Verification items for the finished model (mm, model axes). Face numbers are marked on the shaded views. A direction names the side the tool comes from. Give positions to 0.01 mm unless a question says otherwise; leave off trailing zeros. Order: outer loops, then holes, each group sorted by start corner. A loop starts at its lowest first (then second) coordinate and runs counter-clockwise, first axis right, second up. Notation, with made-up numbers: (-15.75, 32.25) -> (18.25, 32.25) arc R12 cw to (18.25, 39.25) -> close; hole circle Ø2 at (-7.5, -37.75). An arc over 180 degrees is marked (long way). Write each question's results on one line, items separated by ' | '. Start each with the question number.
1. Set-up check for the marked faces 1, 2 and 3: record each of +Z, -Z, +X, -X, +Y, -Y from which the full face is reachable in a straight line by a thin tool's end or side.
2. Cross-section at B-B, the plane x = 0. Enter the section's corners in (y, z).
3. Cross-section at D-D, the plane x = -7.25. Enter the section's corners in (y, z).
4. Depth check by flat-ended pin: pin 1 Ø1.2 at (x, z) = (-5.5, -3.5) entering from +Y; pin 2 Ø4 at (x, y) = (2, 0.5) entering from -Z; pin 3 Ø1 at (x, z) = (-1, -5) entering from -Y. Enter the tip coordinate at first touch or a pass-through.
5. Cross-section at A-A, the plane y = 0. Enter the section's corners in (x, z), then the cut area to 3 significant figures.
6. Mould release check, pull along X, two halves, no side actions. Record for the marked faces 4, 5 and 6: +X half, -X half, draft (parallel to the pull), parting line (faces both ways), or undercut.
7. Material ranges on L1, parallel to Z at x = 7.25, y = -3; L2, parallel to Y at x = -1.75, z = -7.5; L3, parallel to X at y = 0, z = -2.25, recorded low to high. Write a range as from..to.
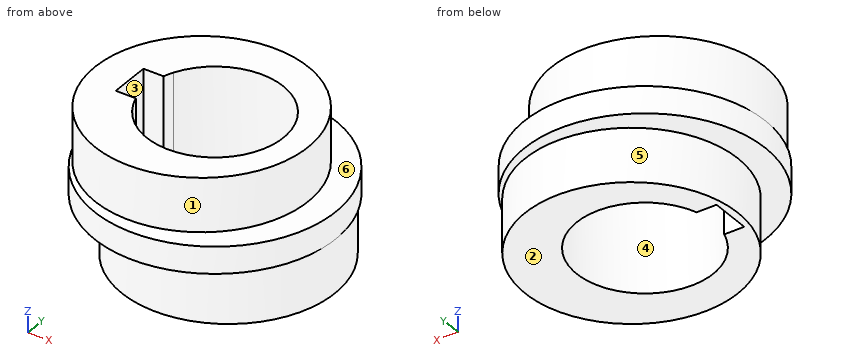
Autodesk Inventor part; units mm, degrees
ref_plane "YZ Plane" through (0, 0, 0) normal (1, 0, 0) x (0, 1, 0)
ref_plane "XZ Plane" through (0, 0, 0) normal (0, 1, 0) x (-1, 0, 0)
ref_plane "XY Plane" through (0, 0, 0) normal (0, 0, 1) x (1, 0, 0)
sketch "Sketch1" plane through (0, 0, 0) normal (0, 0, 1) x (1, 0, 0)
  arc A0 (-4.5, -2.1795) -> (-4.5, 2.1795) centre (0, 0) ccw construction
  line L0 (-4.5, 2.1795) -> (-4.5, -2.1795) construction
  arc A1 (-4.5, 2.1795) -> (-4.5, -2.1795) centre (0, 0) ccw construction
  arc A2 (-4.6, -2.2023) -> (-4.6, 2.2023) centre (0, 0) ccw
  line L1 (-4.6, -2.2023) -> (-4.6, 2.2023)
  circle A3 centre (0, 0) radius 8
  dimension "d0" = 10
  dimension "d1" = 4.359
  dimension "d2" = 0.1
  dimension "d3" = 16
extrude "Extrusion1" add sketch "Sketch1" along normal blind 4
sketch "Sketch2" plane through (0, 0, 0) normal (0, 0, -1) x (-1, 0, 0)
  circle A0 centre (1, 0) radius 7.95
  arc A1 (4.6, 2.2023) -> (4.6, -2.2023) centre (0, 0) ccw
  line L0 (4.6, -2.2023) -> (4.6, 2.2023)
  dimension "d6" = 15.9
  dimension "d7" = 1
extrude "Extrusion2" add sketch "Sketch2" along normal blind 4
sketch "Sketch5" plane through (0, 0, 4) normal (0, 0, 1) x (1, 0, 0)
  circle A0 centre (0, 0) radius 8
extrude "Extrusion5" cut sketch "Sketch5" against normal up to surface (4 mm away)
sketch "Sketch6" plane through (-1, 0, -4) normal (0, 0, -1) x (-1, 0, 0)
  circle A0 centre (-1, 0) radius 9
  arc A1 (3.6, 2.2023) -> (3.6, -2.2023) centre (-1, 0) ccw
  line L0 (3.6, 2.2023) -> (3.6, -2.2023)
  dimension "d19" = 18
extrude "Extrusion6" add sketch "Sketch6" along normal blind 2
sketch "Sketch7" plane through (0, 0, -6) normal (0, 0, -1) x (-1, 0, 0)
  circle A0 centre (-1, 0) radius 7.95
  arc A1 (4.6, 2.2023) -> (4.6, -2.2023) centre (0, 0) ccw
  line L0 (4.6, 2.2023) -> (4.6, -2.2023)
  dimension "d22" = 15.9
  dimension "d23" = 1
extrude "Extrusion7" add sketch "Sketch7" along normal blind 4
sketch "Sketch9" plane through (-1, 0, 0) normal (0, 0, 1) x (1, 0, 0)
  arc A0 (-3.8744, -1.5) -> (-3.8744, 1.5) centre (1, 0) ccw
  arc A1 (-3.6, -2.2023) -> (-3.6, 2.2023) centre (1, 0) ccw construction
  line L0 (-3.8744, 1.5) -> (-5.3744, 1.5)
  line L1 (-5.3744, 1.5) -> (-5.3744, -1.5)
  line L2 (-5.3744, -1.5) -> (-3.8744, -1.5)
  arc A2 (-3.8744, 1.5) -> (-3.8744, -1.5) centre (1, 0) ccw construction
  point P0 (-4.6244, 1.5)
  point P1 (-4.6244, -1.5)
  point P2 (-5.3744, 0)
  dimension "d30" = 3
  dimension "d31" = 1.5
extrude "Extrusion9" cut sketch "Sketch9" against normal through all
properties part number "EccentricBearingShaft" material "Aluminum 6061"
Results below:
1) face 1: +Z | face 2: -Z, +X, -X, +Y, -Y | face 3: +Z, -Z
2) outline: (-9, -6) -> (-7.89, -6) -> (-7.89, -10) -> (-5.1, -10) -> (-5.1, 0) -> (-7.89, 0) -> (-7.89, -4) -> (-9, -4) -> close; (5.1, -10) -> (7.89, -10) -> (7.89, -6) -> (9, -6) -> (9, -4) -> (7.89, -4) -> (7.89, 0) -> (5.1, 0) -> close
3) outline: (-5.33, -6) -> (5.33, -6) -> (5.33, -4) -> (4.91, -4) -> (4.91, 0) -> (-4.91, 0) -> (-4.91, -4) -> (-5.33, -4) -> close
4) pin 1: stops at y = 7.37 | pin 2: passes through | pin 3: stops at y = -8.99
5) outline: (-9, -6) -> (-6.95, -6) -> (-6.95, -10) -> (-6.37, -10) -> (-6.37, 0) -> (-8.95, 0) -> (-8.95, -4) -> (-9, -4) -> close; (5.1, -10) -> (8.95, -10) -> (8.95, -6) -> (9, -6) -> (9, -4) -> (6.95, -4) -> (6.95, 0) -> (5.1, 0) -> close | area: 48.5 mm²
6) face 4: undercut | face 5: parting line | face 6: draft
7) L1: z = -10..-4 | L2: y = -7.46..-4.79, 4.79..7.46 | L3: x = -8.95..-6.37, 5.1..6.95
